from build123d import *

# Parameters (mm, degrees)
F1_DEPTH = 127
F2_R     = 1.5875
F3_DEPTH = 12.7
F4_R     = 1.5875
F5_DEPTH = 12.7


with BuildPart() as f1:
    # F0 (on Top) → F1 (new body)
    with BuildSketch(Plane.XY):
        Polygon((0, 32.662014), (-34.38163, 29.533893), (0, 26.312014), (54.51837, 29.533893), align=None)
    extrude(amount=F1_DEPTH)

    # F2 (on face) → F3 (join)
    with BuildSketch(Plane(origin=(0, 0, 0), x_dir=(1, 0, 0), z_dir=(0, 0, -1))):
        with Locations((0, -29.959638)):
            Circle(F2_R)
    extrude(amount=F3_DEPTH)

    # F4 (on face) → F5 (join)
    with BuildSketch(Plane.XY.offset(127)):
        with Locations((0, 29.418199)):
            Circle(F4_R)
    extrude(amount=F5_DEPTH)


solid = f1.part
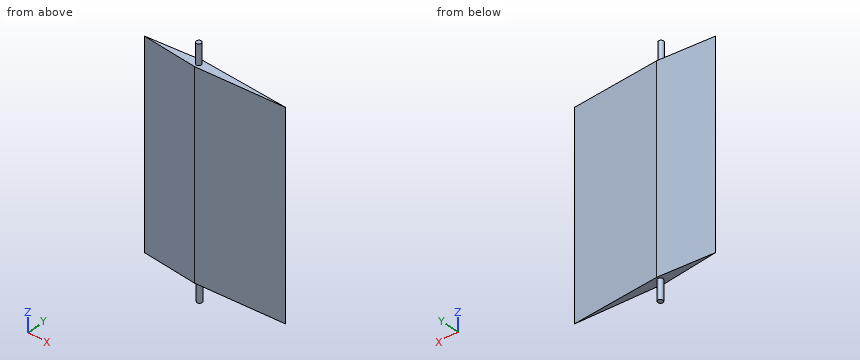
Can you work these out from the model? Positions are in its coordinate system, mm. Coordinates: 2 decimals unless noted, no trailing zeros. Loops run counter-clockwise (first coordinate to the right, second up) from the corner with the lowest first, then second, coordinate; pieces in that order, holes last. Notation, with made-up numbers: M 86,-24.75 L 127,-24.75 A35 cw 127,13.25 Z; hole C 43.5,79 d1. An arc over 180 degrees is marked long. Answer as CSV lines item,"result". Start each with the question number.
1. If I drill on probe 1 along Z at (x, y) = (25.5, 29.5); probe 2 along Y at (x, z) = (-3, 56.5); probe 3 along Y at (x, z) = (46.5, 20), over which ranges is the centre line in solid material (lowest first)? Write a range as [from, to].
2. Suppose I cut it at A-A, the plane z = 20.5. List the corners of the cut face in (x, y) for me, plus the area to 3 significant figures.
3. For pin 1 Ø12 at (x, z) = (32.5, 23.5) entering from +Y; pin 2 Ø1.9 at (x, y) = (17, 29) entering from -Z; pin 3 Ø12 at (x, z) = (39.5, 65) entering from +Y, each with a flat end and sliding along its axis, tell me the tip position at first contact or that it passes through.
4. Suppose I cut it at B-B, the plane x = 49.5. List the corners of the cut face in (y, z) for me, plus the area to 3 significant figures.
Output:
1,probe 1,"z = [0, 127]"
1,probe 2,"y = [26.59, 32.39]"
1,probe 3,"y = [29.06, 29.99]"
2,outline,"M -34.38,29.53 L 0,26.31 L 54.52,29.53 L 0,32.66 Z"
2,area,"282 mm^2"
3,pin 1,"stops at y = 31.14"
3,pin 2,"stops at z = 0"
3,pin 3,"stops at y = 30.74"
4,outline,"M 29.24,0 L 29.82,0 L 29.82,127 L 29.24,127 Z"
4,area,"74.2 mm^2"
